from build123d import *

# Parameters (mm, degrees)
F0_W     = 76.2
F0_H     = 76.2
F0_R     = 24.13
F0_R_2   = 13.97
F1_DEPTH = 6.35
F3_DEPTH = 3.175
F5_DEPTH = 3.175


# Not quite as in the source:
# - after a boolean that leaves OpenCascade's solid faulty, fix() repairs it


with BuildPart() as f1:
    # F0 (on Right) → F1 (new body)
    with BuildSketch(Plane.YZ):
        Rectangle(F0_W, F0_H)
        Circle(F0_R, mode=Mode.SUBTRACT)
        Circle(F0_R)
        Circle(F0_R_2, mode=Mode.SUBTRACT)
        Circle(F0_R_2)
    extrude(amount=F1_DEPTH)

    # F0 (on Right) → F3 (cut)
    with BuildSketch(Plane.YZ):
        Circle(F0_R)
        Circle(F0_R_2, mode=Mode.SUBTRACT)
    extrude(amount=F3_DEPTH, mode=Mode.SUBTRACT)

    # F4 (on face) → F5 (join)
    with BuildSketch(Plane.YZ):
        with BuildLine():
            Line((38.1, 9.5882897328), (38.1, 38.1))
            Line((38.1, 38.1), (10.16, 38.1))
            Line((10.16, 38.1), (10.16, 21.8867836833))
            ThreePointArc((10.16, 21.8867836833), (17.2825787445, 16.8395181624), (22.1432066332, 9.5882897328))
            Line((22.1432066332, 9.5882897328), (38.1, 9.5882897328))
        make_face()
        with BuildLine():
            Line((38.1, -38.1), (38.1, -9.5882897328))
            Line((38.1, -9.5882897328), (22.1432066332, -9.5882897328))
            ThreePointArc((22.1432066332, -9.5882897328), (17.2825787445, -16.8395181624), (10.16, -21.8867836833))
            Line((10.16, -21.8867836833), (10.16, -38.1))
            Line((10.16, -38.1), (38.1, -38.1))
        make_face()
        with BuildLine():
            Line((-10.16, 21.8867836833), (-10.16, 38.1))
            Line((-10.16, 38.1), (-38.1, 38.1))
            Line((-38.1, 38.1), (-38.1, 9.5882897328))
            Line((-38.1, 9.5882897328), (-22.1432066332, 9.5882897328))
            ThreePointArc((-22.1432066332, 9.5882897328), (-17.2825787445, 16.8395181624), (-10.16, 21.8867836833))
        make_face()
        with BuildLine():
            Line((-38.1, -9.5882897328), (-38.1, -38.1))
            Line((-38.1, -38.1), (-10.16, -38.1))
            Line((-10.16, -38.1), (-10.16, -21.8867836833))
            ThreePointArc((-10.16, -21.8867836833), (-17.2825787445, -16.8395181624), (-22.1432066332, -9.5882897328))
            Line((-22.1432066332, -9.5882897328), (-38.1, -9.5882897328))
        make_face()
        with BuildLine():
            Line((36.195, -8.001), (36.195, 8.001))
            Line((36.195, 8.001), (22.7649049855, 8.001))
            ThreePointArc((22.7649049855, 8.001), (24.13, 0), (22.7649049855, -8.001))
            Line((22.7649049855, -8.001), (36.195, -8.001))
        make_face()
        with BuildLine():
            Line((-22.7649049855, 8.001), (-36.195, 8.001))
            Line((-36.195, 8.001), (-36.195, -8.001))
            Line((-36.195, -8.001), (-22.7649049855, -8.001))
            ThreePointArc((-22.7649049855, -8.001), (-24.13, 0), (-22.7649049855, 8.001))
        make_face()
        with BuildLine():
            Line((8.001, 22.7649049855), (8.001, 36.195))
            Line((8.001, 36.195), (-8.001, 36.195))
            Line((-8.001, 36.195), (-8.001, 22.7649049855))
            ThreePointArc((-8.001, 22.7649049855), (0, 24.13), (8.001, 22.7649049855))
        make_face()
        with BuildLine():
            Line((-8.001, -36.195), (8.001, -36.195))
            Line((8.001, -36.195), (8.001, -22.7649049855))
            ThreePointArc((8.001, -22.7649049855), (0, -24.13), (-8.001, -22.7649049855))
            Line((-8.001, -22.7649049855), (-8.001, -36.195))
        make_face()
    extrude(amount=-F5_DEPTH)

    add(f1.part.fix(), mode=Mode.REPLACE)


solid = f1.part
Input: part model. Units: mm. Frame: model coordinates. A direction names the side the tool comes from. Coordinates: 2 decimals unless noted, no trailing zeros. Order: outer loops, then holes, each group sorted by start corner. A loop starts at its lowest first (then second) coordinate and runs counter-clockwise, first axis right, second up. Notation, with made-up numbers: M -39.75,80.5 L 8.25,80.5 A33 ccw 8.25,114.5 Z; hole C 73.25,47.25 d11. An arc over 180 degrees is marked long. One line per question, with ' | ' between items.
Item 1: Section A-A (y = 0). Output: boundary loops of the cut face in (x, z) (3 decimals), then the cut area to 3 significant figures.
Geometry results:
outline: M -3.175,-36.195 L 0,-36.195 L 0,-38.1 L 6.35,-38.1 L 6.35,38.1 L 0,38.1 L 0,36.195 L -3.175,36.195 L -3.175,24.13 L 3.175,24.13 L 3.175,13.97 L 0,13.97 L 0,-13.97 L 3.175,-13.97 L 3.175,-24.13 L -3.175,-24.13 Z | area: 496 mm^2
Item 2: Reachability of faces 1 (the flat face through (2, -1, -38.1)), 2 (the flat face through (-2, -8.001, -29)), 3 (the flat face through (-3.175, 24, -24)), 4 (the flat face through (-2, -30, -8.001)), 5 (the flat face through (3.175, 10, -10)) from +Z, -Z, +X, -X, +Y, -Y: full face, straight path, thin tool, end or side. Return the list, or none.
Geometry results:
face 1: -Z, +X, -X, +Y, -Y | face 2: +Z, -Z, -X | face 3: +Z, -Z, -X, +Y, -Y | face 4: -X, +Y, -Y | face 5: -X
Item 3: Ray query, line 1 along Z through (x, y) = (-1.5, 33.5); line 2 along Z through (x, y) = (2.25, 0); line 3 along Z through (x, y) = (-0.25, 0) (3 decimals). Return the intervals inside material, ascending.
Geometry results:
line 1: z = -38.1 to -9.59, -8 to 8, 9.59 to 38.1 | line 2: z = -38.1 to -24.13, -13.97 to 13.97, 24.13 to 38.1 | line 3: z = -36.195 to -24.13, 24.13 to 36.195
Item 4: Section B-B (x = -1.25). Give the number of separate pieces and of enclosed holes in the cut face, then the cut area to 3 significant figures.
Geometry results:
separate pieces: 8 | enclosed holes: 0 | area: 3,620 mm^2
Item 5: Pin query (flat end, axial travel): pin 1 (3.5 mm diameter, centred on x = -1.5, y = 3, fed in from -Z); pin 2 (1 mm diameter, centred on y = 17, z = -10, fed in from -X) (3 decimals). Return the tip coordinate at first contact, or that it passes through.
Geometry results:
pin 1: stops at z = -38.1 | pin 2: stops at x = 3.175
Item 6: Draft query along Y for faces 6 (the flat face through (-2, 0, 36.195)), 7 (the flat face through (6.35, -1, 1)), 8 (the flat face through (2, -38.1, -1)), 9 (the flat face through (-2, 36.195, 0)). Return one class per face: released by +Y, released by -Y, zero draft, split by the parting line, or undercut.
Geometry results:
face 6: undercut | face 7: zero draft | face 8: released by -Y | face 9: released by +Y
Item 7: Section D-D (z = -21). Output: boundary loops of the cut face in (x, y) (3 decimals), then the cut area to 3 significant figures.
Geometry results:
outline: M -3.175,-38.1 L 6.35,-38.1 L 6.35,38.1 L -3.175,38.1 L -3.175,11.885 L 3.175,11.885 L 3.175,-11.885 L -3.175,-11.885 Z | area: 575 mm^2
